Geometry: final body of the model. Coordinates: model frame, mm. A direction names the side the tool comes from. Give positions to 0.01 mm unless a question says otherwise; leave off trailing zeros. Write each loop counter-clockwise with the first axis right and the second up, starting at its lowest first coordinate (ties: lowest second). Pieces come first, ordered by that corner, then holes. Notation, with made-up numbers: (86, 13) -> (135, 13) arc R11 cw to (135, 26) -> close; hole circle Ø5 at (-12.75, -8). An arc over 180 degrees is marked (long way). Answer in a Markdown table with one row per item. Add a question column.
Item 1: Access query for faces 1 (the flat face through (-960, 10, 1)), 2 (the flat face through (-130, 10, 125)). Directions: +Z, -Z, +X, -X, +Y, -Y. A direction counts if a zero-diameter tool reaches every point of the face in a straight line with its end or side. Return the directions, or none.
Item 2: Section query C-C on z = 113. Output: boundary loops of the cut face in (x, y).
Item 3: Material intervals for probe 1 along X at (y, z) = (1.75, 6); probe 2 along Z at (x, y) = (-633.5, 1); probe 3 along X at (y, z) = (17, 53), sorted ascending. Write a range as from..to.
Item 4: Draft query along X for faces 3 (the flat face through (-487, 20, -2)), 4 (the cylindrical face through (-931.484, 10.14, 114.929)), 5 (the flat face through (-637, 10, 75)). Return one class per face: +X half, -X half, draft (parallel to the pull), parting line (faces both ways), or undercut.
Item 5: Section query B-B on y = 14. Output: boundary loops of the cut face in (x, z).
Item 6: Section query A-A on z = 10. Output: boundary loops of the cut face in (x, y).
Item 7: First-contact query: P1, Ø4, axis at y = 8.5, z = 87.5, coming from the -X side; P2, Ø4, axis at y = 5.5, z = -81, coming from the -X side; P3, Ø1, axis at y = 13, z = 107.5, coming from the -X side. Flat tips, straight axial feed; report the tip coordinate or a pass-through.
```python
from build123d import *

# Parameters (mm, degrees)
SKETCH1_W           = 960
SKETCH1_H           = 290
BOSS_EXTRUDE1_DEPTH = 20
FILLET1_R           = 100
SKETCH5_W           = 20
SKETCH5_H           = 250
SKETCH5_H_2         = 150
CUT_EXTRUDE1_DEPTH  = 20


with BuildPart() as part:
    # Sketch1 → Boss-Extrude1 (new body)
    with BuildSketch(Plane(origin=(0, 0, 0), x_dir=(1, 0, 0), z_dir=(0, 1, 0))):
        with Locations((-480, 0)):
            Rectangle(SKETCH1_W, SKETCH1_H)
    extrude(amount=BOSS_EXTRUDE1_DEPTH)

    # Fillet1
    fillet1_edges = [part.edges().sort_by_distance(p)[0] for p in [
        (-960, 10, 145),
        (-960, 10, -145),
    ]]
    fillet(fillet1_edges, radius=FILLET1_R)

    # Sketch5 → Cut-Extrude1 (cut)
    with BuildSketch(Plane.XZ):
        with Locations((-130, 0)):
            Rectangle(SKETCH5_W, SKETCH5_H)
        with Locations((-637, 0)):
            Rectangle(SKETCH5_W, SKETCH5_H_2)
        with Locations((-837, 0)):
            Rectangle(SKETCH5_W, SKETCH5_H_2)
    extrude(amount=-CUT_EXTRUDE1_DEPTH, mode=Mode.SUBTRACT)


solid = part.part
```
Findings below:
| question | item | result |
|---|---|---|
| 1 | face 1 | +Z, -Z, -X, +Y, -Y |
| 1 | face 2 | +Y, -Y |
| 2 | outline | (-933.32, 0) -> (-140, 0) -> (-140, 20) -> (-933.32, 20) -> close; (-120, 0) -> (0, 0) -> (0, 20) -> (-120, 20) -> close |
| 3 | probe 1 | x = -960..-847, -827..-647, -627..-140, -120..0 |
| 3 | probe 2 | z = -145..-75, 75..145 |
| 3 | probe 3 | x = -959.68..-847, -827..-647, -627..-140, -120..0 |
| 4 | face 3 | draft |
| 4 | face 4 | -X half |
| 4 | face 5 | undercut |
| 5 | outline | (-960, -45) arc R100 ccw to (-860, -145) -> (0, -145) -> (0, 145) -> (-860, 145) arc R100 ccw to (-960, 45) -> close; hole (-847, -75) -> (-827, -75) -> (-827, 75) -> (-847, 75) -> close; hole (-647, -75) -> (-627, -75) -> (-627, 75) -> (-647, 75) -> close; hole (-140, -125) -> (-120, -125) -> (-120, 125) -> (-140, 125) -> close |
| 6 | outline | (-960, 0) -> (-847, 0) -> (-847, 20) -> (-960, 20) -> close; (-827, 0) -> (-647, 0) -> (-647, 20) -> (-827, 20) -> close; (-627, 0) -> (-140, 0) -> (-140, 20) -> (-627, 20) -> close; (-120, 0) -> (0, 0) -> (0, 20) -> (-120, 20) -> close |
| 7 | P1 | stops at x = -951.43 |
| 7 | P2 | stops at x = -954.04 |
| 7 | P3 | stops at x = -938.46 |
